from build123d import *

# Parameters (mm, degrees)
SKETCH_1_W          = 20
SKETCH_1_H          = 13
EXTRUDE_1_DEPTH     = 15
SHELL_1_T           = -1
SKETCH_2_R          = 2.5
SKETCH_2_R_2        = 2
EXTRUDE_4_DEPTH     = 10
SKETCH_3_R          = 4.9
CUT_EXTRUDE_1_DEPTH = 0.2
SKETCH_9_R          = 2.5
SKETCH_9_R_2        = 2
EXTRUDE_8_DEPTH     = 10
SKETCH_6_W          = 2
SKETCH_6_H          = 10
EXTRUDE_10_DEPTH    = 3
SKETCH_10_W         = 2
SKETCH_10_H         = 10
EXTRUDE_11_DEPTH    = 3


with BuildPart() as part:
    # Sketch 1 → Extrude 1 (new body)
    with BuildSketch(Plane.XY):
        Rectangle(SKETCH_1_W, SKETCH_1_H)
    extrude(amount=EXTRUDE_1_DEPTH)

    # Shell 1
    shell_1_openings = [part.faces().sort_by_distance(p)[0] for p in [
        (0, 0, 15),
    ]]
    offset(amount=SHELL_1_T, openings=shell_1_openings, kind=Kind.INTERSECTION)

    # Sketch 3 → Cut-Extrude 1 (cut)
    with BuildSketch(Plane.XY.offset(1)):
        Circle(SKETCH_3_R)
    extrude(amount=-CUT_EXTRUDE_1_DEPTH, mode=Mode.SUBTRACT)

    # Sketch 9 → Extrude 8 (add)
    # profile 1 of 3: a face of its own
    with BuildSketch(Plane(origin=(0, 6.5, 0), x_dir=(1, 0, 0), z_dir=(0, 1, 0))):
        with BuildLine():
            Line((10, -17.5), (10, -15))
            Line((10, -15), (7.5, -15))
            ThreePointArc((7.5, -15), (9.267766953, -15.732233047), (10, -17.5))
        make_face()
    # profile 2 of 3: a face of its own
    with BuildSketch(Plane(origin=(0, 6.5, 0), x_dir=(1, 0, 0), z_dir=(0, 1, 0))):
        with BuildLine():
            Line((10, -20), (10, -17.5))
            ThreePointArc((10, -17.5), (9.267766953, -19.267766953), (7.5, -20))
            Line((7.5, -20), (10, -20))
        make_face()
    # profile 3 of 3: a face of its own
    with BuildSketch(Plane(origin=(0, 6.5, 0), x_dir=(1, 0, 0), z_dir=(0, 1, 0))):
        with Locations((7.5, -17.5)):
            Circle(SKETCH_9_R)
        with Locations(Location((7.5, -17.5, 0), (0, 0, 270))):
            Circle(SKETCH_9_R_2, mode=Mode.SUBTRACT)
    extrude(amount=-EXTRUDE_8_DEPTH)


with BuildPart() as body_2:
    # Sketch 2 → Extrude 4 (new body)
    # profile 1 of 3: a face of its own
    with BuildSketch(Plane(origin=(0, 3.5, 0), x_dir=(1, 0, 0), z_dir=(0, 1, 0))):
        with BuildLine():
            ThreePointArc((-7.5, -20), (-9.267766953, -19.267766953), (-10, -17.5))
            Line((-10, -17.5), (-10, -20))
            Line((-10, -20), (-7.5, -20))
        make_face()
    # profile 2 of 3: a face of its own
    with BuildSketch(Plane(origin=(0, 3.5, 0), x_dir=(1, 0, 0), z_dir=(0, 1, 0))):
        with Locations((-7.5, -17.5)):
            Circle(SKETCH_2_R)
        with Locations(Location((-7.5, -17.5, 0), (0, 0, 270))):
            Circle(SKETCH_2_R_2, mode=Mode.SUBTRACT)
    # profile 3 of 3: a face of its own
    with BuildSketch(Plane(origin=(0, 3.5, 0), x_dir=(1, 0, 0), z_dir=(0, 1, 0))):
        with BuildLine():
            Line((-7.5, -15), (-10, -15))
            Line((-10, -15), (-10, -17.5))
            ThreePointArc((-10, -17.5), (-9.267766953, -15.732233047), (-7.5, -15))
        make_face()
    extrude(amount=-EXTRUDE_4_DEPTH)


    add(part.part)  # Extrude 10 merges part
    # Sketch 6 → Extrude 10 (add)
    with BuildSketch(Plane.ZY.offset(10)):
        with Locations((19, -1.5)):
            Rectangle(SKETCH_6_W, SKETCH_6_H)
    extrude(amount=EXTRUDE_10_DEPTH)

    # Sketch 10 → Extrude 11 (add)
    with BuildSketch(Plane(origin=(10, 0, 0), x_dir=(0, 0, -1), z_dir=(1, 0, 0))):
        with Locations((-19, 1.5)):
            Rectangle(SKETCH_10_W, SKETCH_10_H)
    extrude(amount=EXTRUDE_11_DEPTH)


solid = body_2.part
Here's how the part is built. I have some questions about the finished solid (model axes, mm). A direction names the side the tool comes from. Coordinates: 2 decimals unless noted, no trailing zeros. Write each loop counter-clockwise with the first axis right and the second up, starting at its lowest first coordinate (ties: lowest second). Pieces come first, ordered by that corner, then holes.
Item 1: I want a section at C-C on x = 0. Write out the boundary of the cut face in (y, z).
Item 2: If we mould it in two halves opening along X, with no side actions, what happens to faces 1 (the flat face through (13, 2, 19)), 2 (the flat face through (0, 5.5, 8)), 3 (the flat face through (-11, -2, 18))? For each: +X half, -X half, draft (parallel to the pull), parting line (faces both ways), or undercut.
Item 3: On a 3-axis mill with a long thin cutter (end or side, diameter ignored), from which of +Z, -Z, +X, -X, +Y, -Y can I reach the whole of each face in a straight line? I mean faces 4 (the flat face through (8, 1, 15)), 5 (the flat face through (10, 1, 20)), 6 (the flat face through (-9.8, 3.5, 18)), 7 (the flat face through (0, 0, 0.8)), 8 (the flat face through (9.8, -3.5, 18.1)). Say none if no direction works.
Item 4: I want a section at A-A on z = 17.5. Write out the boundary of the cut face in (x, y), and give its area (3 significant figures).
Item 5: I want a section at B-B on y = 0. Write out the boundary of the cut face in (x, z).
Item 6: I want a section at D-D on z = 5.75. Write out the boundary of the cut face in (x, y), and give its area (3 significant figures).
Item 7: If I drill on line 1 (X direction, y = -2, z = 17.5); line 2 (Y direction, x = 0, z = 0.95); line 3 (Y direction, x = 1.5, z = 3), over which ranges is the centre line in solid material (lowest first)?
Item 8: Will these pins go through, and if not, where does the flat tip stop? pin 1 (5.5 mm diameter, centred on y = -1, z = 4.5, fed in from +X); pin 2 (6 mm diameter, centred on y = 1.5, z = 12.5, fed in from -X); pin 3 (3 mm diameter, centred on x = -1, y = -1, fed in from +Z).
Findings below:
1. outline: (-6.5, 0) - (6.5, 0) - (6.5, 15) - (5.5, 15) - (5.5, 1) - (4.9, 1) - (4.9, 0.8) - (-4.9, 0.8) - (-4.9, 1) - (-5.5, 1) - (-5.5, 15) - (-6.5, 15) - close
2. face 1: +X half
2. face 2: undercut
2. face 3: draft
3. face 4: none
3. face 5: +Z, +X, -X, +Y, -Y
3. face 6: +Z, -X, +Y
3. face 7: +Z
3. face 8: +Z, +X, -Y
4. outline: (-10, -6.5) - (-9.5, -6.5) - (-9.5, 3.5) - (-10, 3.5) - close; (-5.5, -6.5) - (-5, -6.5) - (-5, 3.5) - (-5.5, 3.5) - close; (5, -3.5) - (5.5, -3.5) - (5.5, 6.5) - (5, 6.5) - close; (9.5, -3.5) - (10, -3.5) - (10, 6.5) - (9.5, 6.5) - close
4. area: 20.0 mm2
5. outline: (-13, 18) - (-10, 18) - (-10, 0) - (10, 0) - (10, 18) - (13, 18) - (13, 20) - (7.5, 20) arc R2.5 ccw to (7.5, 15) - (9, 15) - (9, 1) - (4.9, 1) - (4.9, 0.8) - (-4.9, 0.8) - (-4.9, 1) - (-9, 1) - (-9, 15) - (-7.5, 15) arc R2.5 ccw to (-7.5, 20) - (-13, 20) - close; hole circle Ø4 at (-7.5, 17.5); hole circle Ø4 at (7.5, 17.5)
6. outline: (-10, -6.5) - (10, -6.5) - (10, 6.5) - (-10, 6.5) - close; hole (-9, -5.5) - (9, -5.5) - (9, 5.5) - (-9, 5.5) - close
6. area: 62.0 mm2
7. line 1: x = -10 to -9.5, -5.5 to -5, 5 to 5.5, 9.5 to 10
7. line 2: y = -6.5 to -4.9, 4.9 to 6.5
7. line 3: y = -6.5 to -5.5, 5.5 to 6.5
8. pin 1: stops at x = 10
8. pin 2: stops at x = -10
8. pin 3: stops at z = 0.8
